Geometry: final body of the model. Coordinates: model frame, mm. A direction names the side the tool comes from. Coordinates: 2 decimals unless noted, no trailing zeros. Order: outer loops, then holes, each group sorted by start corner. A loop starts at its lowest first (then second) coordinate and runs counter-clockwise, first axis right, second up. Notation, with made-up numbers: M 69.25,79.5 L 107.25,79.5 A21 cw 107.25,112.5 Z; hole C 50.5,47 d8. An arc over 180 degrees is marked long. One line per question, with ' | ' between items.
from build123d import *

# Parameters (mm, degrees)
SKETCH1_W           = 23
SKETCH1_H           = 7
SKETCH1_W_2         = 6
SKETCH1_H_2         = 17
BOSS_EXTRUDE1_DEPTH = 2.5
BOSS_EXTRUDE2_DEPTH = 2.5


with BuildPart() as part:
    # Sketch1 → Boss-Extrude1 (new body)
    with BuildSketch(Plane(origin=(0, 0, 0), x_dir=(1, 0, 0), z_dir=(0, 1, 0))):
        with BuildLine():
            Line((-26.5, 8), (-26.5, -8))
            ThreePointArc((-26.5, -8), (-22.399494937, -17.899494937), (-12.5, -22))
            Line((-12.5, -22), (12.5, -22))
            ThreePointArc((12.5, -22), (22.399494937, -17.899494937), (26.5, -8))
            Line((26.5, -8), (26.5, 8))
            ThreePointArc((26.5, 8), (22.399494937, 17.899494937), (12.5, 22))
            Line((12.5, 22), (-12.5, 22))
            ThreePointArc((-12.5, 22), (-22.399494937, 17.899494937), (-26.5, 8))
        make_face()
        with Locations((0, -15.5)):
            Rectangle(SKETCH1_W, SKETCH1_H, mode=Mode.SUBTRACT)
        with Locations((20, 0)):
            Rectangle(SKETCH1_W_2, SKETCH1_H_2, mode=Mode.SUBTRACT)
        with Locations((0, 15.5)):
            Rectangle(SKETCH1_W, SKETCH1_H, mode=Mode.SUBTRACT)
    extrude(amount=BOSS_EXTRUDE1_DEPTH)

    # Sketch2 → Boss-Extrude2 (add)
    with BuildSketch(Plane.XZ):
        with BuildLine():
            Line((-17, 15.794228634), (-18.25, 17.959292144))
            ThreePointArc((-18.25, 17.959292144), (-21.623563413, 15.000756434), (-23.608147002, 10.976419019))
            Line((-23.608147002, 10.976419019), (-21.193332437, 10.329371406))
            ThreePointArc((-21.193332437, 10.329371406), (-19.640180063, 13.478852861), (-17, 15.794228634))
        make_face()
        with BuildLine():
            Line((23.608147002, 10.976419019), (21.193332437, 10.329371406))
            ThreePointArc((21.193332437, 10.329371406), (19.640180063, 13.478852861), (17, 15.794228634))
            Line((17, 15.794228634), (18.25, 17.959292144))
            ThreePointArc((18.25, 17.959292144), (21.623563413, 15.000756434), (23.608147002, 10.976419019))
        make_face()
        with BuildLine():
            Line((17, -15.794228634), (18.25, -17.959292144))
            ThreePointArc((18.25, -17.959292144), (21.623563413, -15.000756434), (23.608147002, -10.976419019))
            Line((23.608147002, -10.976419019), (21.193332437, -10.329371406))
            ThreePointArc((21.193332437, -10.329371406), (19.640180063, -13.478852861), (17, -15.794228634))
        make_face()
        with BuildLine():
            Line((-23.608147002, -10.976419019), (-21.193332437, -10.329371406))
            ThreePointArc((-21.193332437, -10.329371406), (-19.640180063, -13.478852861), (-17, -15.794228634))
            Line((-17, -15.794228634), (-18.25, -17.959292144))
            ThreePointArc((-18.25, -17.959292144), (-21.623563413, -15.000756434), (-23.608147002, -10.976419019))
        make_face()
    extrude(amount=BOSS_EXTRUDE2_DEPTH)


solid = part.part
1. Section C-C, the plane z = -4. Output: boundary loops of the cut face in (x, y).
Response values:
outline: M -26.5,0 L 17,0 L 17,2.5 L -26.5,2.5 Z; M 23,0 L 26.5,0 L 26.5,2.5 L 23,2.5 Z
2. Section D-D, the plane x = 20. Output: boundary loops of the cut face in (y, z), and give its area (3 significant figures).
Response values:
outline: M -2.5,-16.72 L 0,-16.72 L 0,-19.82 L 2.5,-19.82 L 2.5,-8.5 L 0,-8.5 L 0,-12.97 L -2.5,-12.97 Z; M -2.5,12.97 L 0,12.97 L 0,8.5 L 2.5,8.5 L 2.5,19.82 L 0,19.82 L 0,16.72 L -2.5,16.72 Z | area: 75.3 mm^2
3. Section B-B, the plane x = -6.5. Output: boundary loops of the cut face in (y, z).
Response values:
outline: M 0,-22 L 2.5,-22 L 2.5,-19 L 0,-19 Z; M 0,-12 L 2.5,-12 L 2.5,12 L 0,12 Z; M 0,19 L 2.5,19 L 2.5,22 L 0,22 Z
4. Section A-A, the plane y = -1.3. Output: boundary loops of the cut face in (x, z).
Response values:
outline: M -23.61,-10.98 A11.5 ccw -18.25,-17.96 L -17,-15.79 A9 cw -21.19,-10.33 Z; M -23.61,10.98 L -21.19,10.33 A9 cw -17,15.79 L -18.25,17.96 A11.5 ccw Z; M 17,-15.79 L 18.25,-17.96 A11.5 ccw 23.61,-10.98 L 21.19,-10.33 A9 cw Z; M 17,15.79 A9 cw 21.19,10.33 L 23.61,10.98 A11.5 ccw 18.25,17.96 Z
5. Material intervals for line 1 (Z direction, x = 6.5, y = 2.2); line 2 (X direction, y = 1.35, z = -0.5); line 3 (Y direction, x = -8.5, z = -2.5), sorted ascending. Write a range as [from, to].
Response values:
line 1: z = [-22, -19], [-12, 12], [19, 22] | line 2: x = [-26.5, 17], [23, 26.5] | line 3: y = [0, 2.5]
6. Draft query along X for faces 1 (the face through (11.5, 1, 16)), 2 (the face through (0, 1, 22)), 3 (the face through (22.42, -1.23, -10.66)). Return one class per face: pulls with the +X half, pulls with the -X half, needs draft (parallel to the pull), parting line crosses it, or undercut.
Response values:
face 1: undercut | face 2: needs draft | face 3: pulls with the +X half
7. Pin query (flat end, axial travel): P1, Ø1.5, axis at x = -14.5, z = 16.5, coming from the -Y side; P2, Ø0.8, axis at y = 1.5, z = 14, coming from the -X side; P3, Ø0.8, axis at y = 2, z = -14, coming from the +X side. Return the tip coordinate at first contact, or that it passes through.
Response values:
P1: stops at y = 0 | P2: stops at x = -25.33 | P3: stops at x = 25.33
8. Access query for faces 4 (the face through (-21.585, -1.232, -15.051)), 5 (the face through (17.616, -1.232, 16.862)), 6 (the face through (19.7, -1.2, -13.4)), 7 (the face through (17.616, -1.232, -16.862)), 8 (the face through (23, 1, 0)). Directions: +Z, -Z, +X, -X, +Y, -Y. A direction counts if a zero-diameter tool reaches every point of the face in a straight line with its end or side. Return the directions, or none.
Response values:
face 4: -Z, -X, -Y | face 5: +Z, -Y | face 6: -Y | face 7: -Z, -Y | face 8: +Y, -Y
